Work out the finished part from the listing and answer in its coordinate system (mm). Face numbers are marked on the shaded views. A direction names the side the tool comes from. Round coordinates to 2 decimals unless told otherwise and drop trailing zeros. Order: outer loops, then holes, each group sorted by start corner. A loop starts at its lowest first (then second) coordinate and runs counter-clockwise, first axis right, second up. Notation, with made-up numbers: (16.5, 73) - (67.5, 73) arc R8 ccw to (67.5, 88) - close; hole circle Ø6 at (56, 7.25). An arc over 180 degrees is marked (long way). Answer in a Markdown table with one row per item.
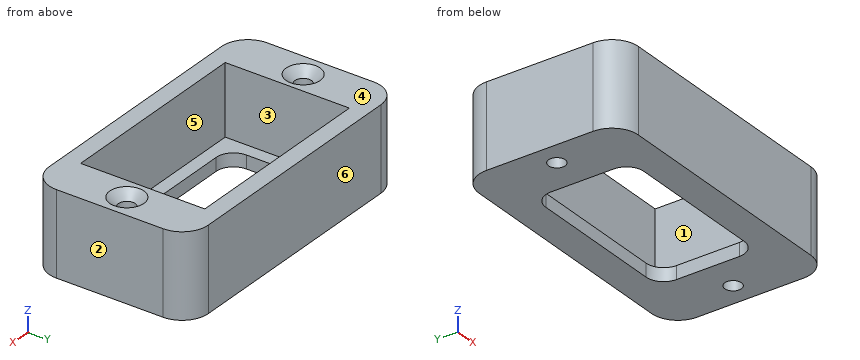
from build123d import *

# Parameters (mm, degrees)
SKETCH_W      = 33.2
SKETCH_H      = 18.2
SKETCH_R      = 0.95
SKETCH_W_2    = 22.8
SKETCH_H_2    = 14.2
PAD_DEPTH     = 9.5
SKETCH001_W   = 22.8
SKETCH001_H   = 14.2
SKETCH001_W_2 = 19.8
SKETCH001_H_2 = 11.2
PAD001_DEPTH  = 1.5
CHAMFER_SIZE  = 1
FILLET_R      = 2
FILLET001_R   = 3


with BuildPart() as part:
    # Sketch → Pad (new body)
    with BuildSketch(Plane.XY):
        Rectangle(SKETCH_W, SKETCH_H)
        with Locations((-13.9, 0)):
            Circle(SKETCH_R, mode=Mode.SUBTRACT)
        with Locations((13.9, 0)):
            Circle(SKETCH_R, mode=Mode.SUBTRACT)
        Rectangle(SKETCH_W_2, SKETCH_H_2, mode=Mode.SUBTRACT)
    extrude(amount=PAD_DEPTH)

    # Sketch001 (on Face11 of Pad) → Pad001 (join)
    with BuildSketch(Plane(origin=(0, 0, 0), x_dir=(1, 0, 0), z_dir=(0, 0, -1))):
        Rectangle(SKETCH001_W, SKETCH001_H)
        Rectangle(SKETCH001_W_2, SKETCH001_H_2, mode=Mode.SUBTRACT)
    extrude(amount=-PAD001_DEPTH)

    # Chamfer
    chamfer_edges = [part.edges().sort_by_distance(p)[0] for p in [
        (12.95, 0, 9.5),
        (-14.85, 0, 9.5),
    ]]
    chamfer(chamfer_edges, length=CHAMFER_SIZE)

    # Fillet
    fillet_edges = [part.edges().sort_by_distance(p)[0] for p in [
        (9.9, -5.6, 0.75),
        (-9.9, -5.6, 0.75),
        (-9.9, 5.6, 0.75),
        (9.9, 5.6, 0.75),
    ]]
    fillet(fillet_edges, radius=FILLET_R)

    # Fillet001
    fillet001_edges = [part.edges().sort_by_distance(p)[0] for p in [
        (16.6, 9.1, 4.75),
        (-16.6, 9.1, 4.75),
        (16.6, -9.1, 4.75),
        (-16.6, -9.1, 4.75),
    ]]
    fillet(fillet001_edges, radius=FILLET001_R)


solid = part.part
1) This flat-tipped pin is pushed along its axis until it touches: pin 1 (1.1 mm diameter, centred on x = 13.9, y = 0, fed in from -Z). Where does it stop, or does it pass through?
Filled in:
| item | result |
|---|---|
| pin 1 | passes through |
2) Which of the six approach directions +Z, -Z, +X, -X, +Y, -Y give full straight-line access (tool end or side, diameter ignored) to the marked faces 1 and 2?
Filled in:
| item | result |
|---|---|
| face 1 | +Z |
| face 2 | +Z, -Z, +X, +Y, -Y |
3) Find the intervals of material crossed by probe 1 along Y at (x, z) = (10, 8.75); probe 2 along X at (y, z) = (4.75, 8.25); probe 3 along Y at (x, z) = (3, 1), in increasing order. Write a range as from..to.
Filled in:
| item | result |
|---|---|
| probe 1 | y = -9.1..-7.1, 7.1..9.1 |
| probe 2 | x = -16.6..-11.4, 11.4..16.6 |
| probe 3 | y = -9.1..-5.6, 5.6..9.1 |
4) Find section D-D, the plane y = 0. Give the vertices of the cut face in (x, z), then the cut area to 3 significant figures.
Filled in:
| item | result |
|---|---|
| outline | (-16.6, 0) - (-14.85, 0) - (-14.85, 8.5) - (-15.85, 9.5) - (-16.6, 9.5) - close; (-12.95, 0) - (-9.9, 0) - (-9.9, 1.5) - (-11.4, 1.5) - (-11.4, 9.5) - (-11.95, 9.5) - (-12.95, 8.5) - close; (9.9, 0) - (12.95, 0) - (12.95, 8.5) - (11.95, 9.5) - (11.4, 9.5) - (11.4, 1.5) - (9.9, 1.5) - close; (14.85, 0) - (16.6, 0) - (16.6, 9.5) - (15.85, 9.5) - (14.85, 8.5) - close |
| area | 65.2 mm^2 |
5) Find section A-A, the plane x = -6.5. Give the vertices of the cut face in (y, z).
Filled in:
| item | result |
|---|---|
| outline | (-9.1, 0) - (-5.6, 0) - (-5.6, 1.5) - (-7.1, 1.5) - (-7.1, 9.5) - (-9.1, 9.5) - close; (5.6, 0) - (9.1, 0) - (9.1, 9.5) - (7.1, 9.5) - (7.1, 1.5) - (5.6, 1.5) - close |
6) The mould has two halves that part along Y. Classify the marked faces 3, 4, 5 and 6: released by +Y, released by -Y, zero draft, split by the parting line, or undercut.
Filled in:
| item | result |
|---|---|
| face 3 | undercut |
| face 4 | zero draft |
| face 5 | undercut |
| face 6 | released by +Y |
7) Find section B-B, the plane y = -2.5. Give the vertices of the cut face in (x, z), then the cut area to 3 significant figures.
Filled in:
| item | result |
|---|---|
| outline | (-16.6, 0) - (-9.9, 0) - (-9.9, 1.5) - (-11.4, 1.5) - (-11.4, 9.5) - (-16.6, 9.5) - close; (9.9, 0) - (16.6, 0) - (16.6, 9.5) - (11.4, 9.5) - (11.4, 1.5) - (9.9, 1.5) - close |
| area | 103 mm^2 |
8) Find section C-C, the plane z = 3.25. Give the vertices of the cut face in (x, y), then the cut area to 3 significant figures.
Filled in:
| item | result |
|---|---|
| outline | (-16.6, -6.1) arc R3 ccw to (-13.6, -9.1) - (13.6, -9.1) arc R3 ccw to (16.6, -6.1) - (16.6, 6.1) arc R3 ccw to (13.6, 9.1) - (-13.6, 9.1) arc R3 ccw to (-16.6, 6.1) - close; hole circle Ø1.9 at (-13.9, 0); hole (-11.4, -7.1) - (11.4, -7.1) - (11.4, 7.1) - (-11.4, 7.1) - close; hole circle Ø1.9 at (13.9, 0) |
| area | 267 mm^2 |
